Autodesk Inventor part; units mm, degrees
ref_plane "YZ Plane" through (0, 0, 0) normal (1, 0, 0) x (0, 1, 0)
ref_plane "XZ Plane" through (0, 0, 0) normal (0, 1, 0) x (-1, 0, 0)
ref_plane "XY Plane" through (0, 0, 0) normal (0, 0, 1) x (1, 0, 0)
sketch "Sketch1" plane through (0, 0, 0) normal (0, 0, 1) x (1, 0, 0)
  line L0 (-3.3401, -3.4417) -> (3.3401, -3.4417)
  line L1 (3.3401, -3.4417) -> (3.3401, 1.1557)
  line L2 (1.0541, 3.4417) -> (-1.0541, 3.4417)
  line L3 (-3.3401, 1.1557) -> (-3.3401, -3.4417)
  line L4 (-3.3401, -3.4417) -> (3.3401, 3.4417) construction
  line L5 (3.3401, -3.4417) -> (-3.3401, 3.4417) construction
  arc A0 (-1.0541, 3.4417) -> (-3.3401, 1.1557) centre (-1.0541, 1.1557) ccw
  arc A1 (3.3401, 1.1557) -> (1.0541, 3.4417) centre (1.0541, 1.1557) ccw
  point P0 (0, 0)
  dimension "d0" = 6.6802
  dimension "d1" = 6.8834
  dimension "d2" = 2.286
extrude "Extrusion1" add sketch "Sketch1" along normal blind 2.54
sketch "Sketch2" plane through (0, 0, 2.54) normal (0, 0, 1) x (1, 0, 0)
  circle A0 centre (0, 0) radius 3.0734
  dimension "d5" = 6.1468
extrude "Extrusion2" cut sketch "Sketch2" against normal blind 0.127
sketch "Sketch4" plane through (0, 0, 2.413) normal (0, 0, 1) x (1, 0, 0)
  circle A0 centre (0, 0) radius 3.0734
  arc A1 (-1.9656, 0.4168) -> (1.9656, 0.4168) centre (0, 0) ccw
  arc A2 (-1.3084, 0.2505) -> (1.3084, 0.2505) centre (0, 0) ccw
  circle A3 centre (1.6419, 0.3144) radius 0.3175
  line L0 (0, 0) -> (0, 0.9465)
  arc A4 (1.9656, 0.4168) -> (1.3084, 0.2505) centre (1.6419, 0.3144) ccw
  arc A5 (-1.3084, 0.2505) -> (-1.9656, 0.4168) centre (-1.6419, 0.3144) ccw
  dimension "d8" = 0.6772
extrude "Extrusion3" cut sketch "Sketch4" against normal blind 0.508 contours A5 A2 A4 A1
sketch "Sketch5" plane through (1.6419, 0.3144, 2.413) normal (0, 0, 1) x (1, 0, 0)
  circle A0 centre (0, 0) radius 0.3175
  point P0 (-1.6419, -0.3144)
extrude "Extrusion4" cut sketch "Sketch5" against normal blind 0.508
sketch "Sketch6" plane through (0, 0, 0) normal (0, 0, -1) x (-1, 0, 0)
  line L0 (3.3401, 1.1557) -> (3.3401, -3.4417)
  line L1 (-1.0541, 3.4417) -> (1.0541, 3.4417)
  line L2 (-3.3401, -3.4417) -> (-3.3401, 1.1557)
  line L3 (-1.905, -1.0033) -> (1.905, -1.0033)
  line L4 (1.905, -1.0033) -> (1.905, 2.8067)
  line L5 (1.905, 2.8067) -> (-1.905, 2.8067)
  line L6 (-1.905, 2.8067) -> (-1.905, -1.0033)
  point P0 (0, 0)
  dimension "d13" = 3.81
  dimension "d14" = 3.81
  dimension "d15" = 6.6802
  dimension "d16" = 1.4351
  dimension "d17" = 0.635
extrude "Extrusion5" cut sketch "Sketch6" against normal blind 0.381
equation "\"d16\" = -0.5 * d13 + 0.5 * d15"
properties part number "trim pot_ body"
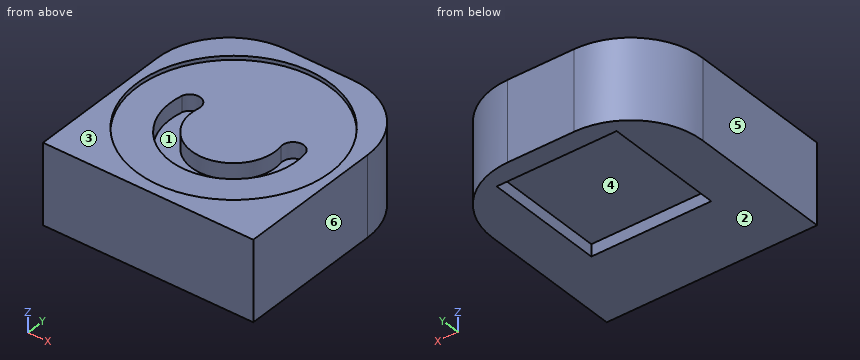
CAD build for the part. Positions are in the model's coordinates, mm. Face numbers are marked on the shaded views. A direction names the side the tool comes from. Round coordinates to 2 decimals unless told otherwise and drop trailing zeros. Order: outer loops, then holes, each group sorted by start corner. A loop starts at its lowest first (then second) coordinate and runs counter-clockwise, first axis right, second up. Notation, with made-up numbers: (18, 69.5) - (67, 69.5) arc R16 cw to (67, 76.5) - close; hole circle Ø4 at (85, -30.5). An arc over 180 degrees is marked (long way). Answer as CSV lines item,"result". Start each with the question number.
1. Saw through at A-A, the plane z = 0.3. Write the cut outline in (x, y) (3 decimals).
2. Pin check, flat tips, straight feed: pin 1 (3 mm diameter, centred on x = -0.5, y = -0.5, fed in from +Z); pin 2 (1.1 mm diameter, centred on x = -0.5, y = 1, fed in from -Z). Stop position of each tip, or through.
3. Pull direction X, two halves, no side cores. Call the marked faces 3, 4, 5 and 6: +X half, -X half, draft (parallel to the pull), parting line (faces both ways), or undercut.
4. Drill centre lines: L1, parallel to X at y = 0, z = 2.35; L2, parallel to Z at x = -1.25, y = 1.5; L3, parallel to Y at x = -0.75, z = 2.15. Where is each one in solid material? Low to high. Write a range as [from, to].
5. Saw through at D-D, the plane z = 1.3. Write the cut outline in (x, y).
6. Saw through at B-B, the plane x = 0. Write the cut outline in (y, z) (3 decimals).
7. Tool access for the marked faces 1 and 2: list every direction of +Z, -Z, +X, -X, +Y, -Y with a clear straight run to the whole face (end or side of a thin tool).
Model answer:
1,outline,"(-3.34, -3.442) - (3.34, -3.442) - (3.34, 1.156) arc R2.286 ccw to (1.054, 3.442) - (-1.054, 3.442) arc R2.286 ccw to (-3.34, 1.156) - close; hole (-1.905, -1.003) - (1.905, -1.003) - (1.905, 2.807) - (-1.905, 2.807) - close"
2,pin 1,"stops at z = 2.41"
2,pin 2,"stops at z = 0.38"
3,face 3,"draft"
3,face 4,"undercut"
3,face 5,"-X half"
3,face 6,"+X half"
4,L1,"x = [-3.34, -2.01], [-1.33, 1.33], [2.01, 3.34]"
4,L2,"z = [0.38, 2.41]"
4,L3,"y = [-3.44, -1.86], [-1.1, 3.44]"
5,outline,"(-3.34, -3.44) - (3.34, -3.44) - (3.34, 1.16) arc R2.29 ccw to (1.05, 3.44) - (-1.05, 3.44) arc R2.29 ccw to (-3.34, 1.16) - close"
6,outline,"(-3.442, 0) - (-1.003, 0) - (-1.003, 0.381) - (2.807, 0.381) - (2.807, 0) - (3.442, 0) - (3.442, 2.54) - (3.073, 2.54) - (3.073, 2.413) - (-1.332, 2.413) - (-1.332, 1.905) - (-2.009, 1.905) - (-2.009, 2.413) - (-3.073, 2.413) - (-3.073, 2.54) - (-3.442, 2.54) - close"
7,face 1,"+Z"
7,face 2,"-Z, +X, -X, +Y, -Y"
